```python
from build123d import *

# Parameters (mm, degrees)
PAD007_DEPTH    = 2
PAD008_DEPTH    = 1
SKETCH021_W     = 20.3
SKETCH021_H     = 23.4
POCKET008_DEPTH = 0.6
PAD009_DEPTH    = 3
SKETCH024_W     = 7.2
SKETCH024_H     = 1.2
POCKET010_DEPTH = 1.2
FILLET002_R     = 0.9


with BuildPart() as part:
    # Sketch019 → Pad007 (new body)
    with BuildSketch(Plane.XY):
        with BuildLine():
            Line((-13.864971, -3.085), (14.264998, -3.085))
            ThreePointArc((14.264998, -3.085), (18.224807, -1.444793), (19.865014, 2.515016))
            Line((19.865014, 2.515016), (19.865014, 23.284984))
            ThreePointArc((19.865014, 23.284984), (18.224807, 27.244793), (14.264998, 28.885))
            Line((14.264998, 28.885), (-13.864971, 28.885))
            ThreePointArc((-13.864971, 28.885), (-17.82478, 27.244793), (-19.464986, 23.284984))
            Line((-19.464986, 23.284984), (-19.464986, 2.515016))
            ThreePointArc((-19.464986, 2.515016), (-17.82478, -1.444793), (-13.864971, -3.085))
        make_face()
        with BuildLine():
            Line((-18.464986, 23.284984), (-18.464986, 2.515016))
            ThreePointArc((-18.464986, 2.515016), (-17.117673, -0.737687), (-13.864971, -2.085))
            Line((-13.864971, -2.085), (14.264998, -2.085))
            ThreePointArc((14.264998, -2.085), (17.5177, -0.737687), (18.865014, 2.515016))
            Line((18.865014, 2.515016), (18.865014, 23.284984))
            ThreePointArc((18.865014, 23.284984), (17.5177, 26.537687), (14.264998, 27.885))
            Line((14.264998, 27.885), (-13.864971, 27.885))
            ThreePointArc((-13.864971, 27.885), (-17.117673, 26.537687), (-18.464986, 23.284984))
        make_face(mode=Mode.SUBTRACT)
    extrude(amount=PAD007_DEPTH)

    # Sketch020 → Pad008 (join)
    with BuildSketch(Plane.XY):
        with BuildLine():
            Line((-20.964986, 23.284984), (-20.964986, 2.515016))
            ThreePointArc((-20.964986, 2.515016), (-18.88544, -2.505454), (-13.864971, -4.585))
            Line((-13.864971, -4.585), (14.264998, -4.585))
            ThreePointArc((14.264998, -4.585), (19.285467, -2.505454), (21.365014, 2.515016))
            Line((21.365014, 2.515016), (21.365014, 23.284984))
            ThreePointArc((21.365014, 23.284984), (19.285467, 28.305454), (14.264998, 30.385))
            Line((14.264998, 30.385), (-13.864971, 30.385))
            ThreePointArc((-13.864971, 30.385), (-18.88544, 28.305454), (-20.964986, 23.284984))
        make_face()
    extrude(amount=-PAD008_DEPTH)

    # Sketch021 → Pocket008 (cut)
    with BuildSketch(Plane.XY):
        with Locations((8.55, 12.7)):
            Rectangle(SKETCH021_W, SKETCH021_H)
    extrude(amount=-POCKET008_DEPTH, mode=Mode.SUBTRACT)

    # Sketch023 → Pad009 (join)
    with BuildSketch(Plane.XZ):
        Polygon((-13.864971, 0), (14.264998, 0), (14.264998, 8.25), (12.364998, 8.25), (12.364998, 4.75), (6.164998, 4.75), (6.164998, 8.25), (3.1, 8.25), (3.1, 4.75), (-3.1, 4.75), (-3.1, 8.25), (-5.764971, 8.25), (-5.764971, 4.75), (-11.964971, 4.75), (-11.964971, 8.25), (-13.864971, 8.25), align=None)
    extrude(amount=PAD009_DEPTH)

    # Sketch024 → Pocket010 (cut)
    with BuildSketch(Plane.XZ):
        with Locations((-8.864971, 6.5)):
            Rectangle(SKETCH024_W, SKETCH024_H)
        with Locations((0, 6.5)):
            Rectangle(SKETCH024_W, SKETCH024_H)
        with Locations((9.264998, 6.5)):
            Rectangle(SKETCH024_W, SKETCH024_H)
    extrude(amount=POCKET010_DEPTH, mode=Mode.SUBTRACT)

    # Fillet002
    fillet002_edges = [part.edges().sort_by_distance(p)[0] for p in [
        (-20.964986, 12.9, -1),
        (-18.88544, 28.305454, -1),
        (0.200014, 30.385, -1),
        (19.285467, 28.305454, -1),
        (21.365014, 12.9, -1),
        (19.285467, -2.505454, -1),
        (0.200014, -4.585, -1),
        (-18.88544, -2.505454, -1),
    ]]
    fillet(fillet002_edges, radius=FILLET002_R)


with BuildPart() as part_1:
    # Body004 placement: moved
    add(part.part.moved(Location((0, 0, 0.9))))


solid = part_1.part
```
The listing builds one solid part. Answer for the finished solid, in the listing's coordinates (mm). A direction names the side the tool comes from. Coordinates: 2 decimals unless noted, no trailing zeros. Loops run counter-clockwise (first coordinate to the right, second up) from the corner with the lowest first, then second, coordinate; pieces in that order, holes last. Notation, with made-up numbers: (73.25, 8.25) -> (104.25, 8.25) arc R19 ccw to (104.25, 44.25) -> close; hole circle Ø1 at (-25.5, 3). An arc over 180 degrees is marked (long way). Return JSON: item names as keys, results as strings. Group by question number.
(1) A cutting plane is placed at D-D on z = 5. Write down the section's boundary in (x, y) (3 decimals), and give its area (3 significant figures).
(2) Find the intervals of material crossed by probe 1 along X at (y, z) = (18, 1.75); probe 2 along X at (y, z) = (-1, 2.25) (3 decimals); probe 3 along Z at (x, y) = (10.5, 25), in increasing order. Write a range as from..to.
(3) A cutting plane is placed at B-B on z = 2. Write down the section's boundary in (x, y) (3 decimals), and give its area (3 significant figures).
(4) A cutting plane is placed at A-A on y = 4. Write down the section's boundary in (x, z), and give its area (3 significant figures).
(5) Which of the six approach directions +Z, -Z, +X, -X, +Y, -Y give full straight-line access (tool end or side, diameter ignored) to faces 1 (the flat face through (0, -3, 5)), 2 (the flat face through (19.865, 13, 2)), 3 (the flat face through (0, -4, 0.9)), 4 (the cylindrical face through (18.18, -1.49, 1.89))?
(6) Determine the mould class of faces 5 (the flat face through (-5.265, -1, 7)), 6 (the cylindrical face through (0.4, -4.33, 0.17)), 7 (the flat face through (3.6, -1, 7)), 8 (the cylindrical face through (-17.87, -1.4, 1.89)) for opening direction X: released by +X, released by -X, zero draft, split by the parting line, or undercut.
(7) A cutting plane is placed at C-C on x = -6.5. Write down the section's boundary in (y, z) (3 decimals).
(8) Given pin 1 Ø1.3 at (y, z) = (-1, 7.5) entering from +X (3 decimals); pin 2 Ø4 at (x, z) = (12.5, 8) entering from -Y; pin 3 Ø2 at (y, z) = (8, 2) entering from -X (3 decimals); pin 4 Ø0.6 at (x, y) = (-3, -0.5) entering from +Z, each flat-ended and moving along its own axis, determine where each tip first touches the part or whether it passes through.
The answers:
{
 "1": {"outline": "(-13.865, -3) -> (14.265, -3) -> (14.265, 0) -> (-13.865, 0) -> close", "area": "84.4 mm^2"},
 "2": {"probe 1": "x = -19.46..-18.46, 18.87..19.87", "probe 2": "x = -18.224..-16.832, -13.865..14.265, 17.232..18.624", "probe 3": "z = -0.1..0.9"},
 "3": {"outline": "(-19.465, 2.515) arc R5.6 ccw to (-13.865, -3.085) -> (14.265, -3.085) arc R5.6 ccw to (19.865, 2.515) -> (19.865, 23.285) arc R5.6 ccw to (14.265, 28.885) -> (-13.865, 28.885) arc R5.6 ccw to (-19.465, 23.285) -> close; hole (-18.465, 2.515) arc R4.6 ccw to (-13.865, -2.085) -> (-13.865, 0) -> (14.265, 0) -> (14.265, -2.085) arc R4.6 ccw to (18.865, 2.515) -> (18.865, 23.285) arc R4.6 ccw to (14.265, 27.885) -> (-13.865, 27.885) arc R4.6 ccw to (-18.465, 23.285) -> close", "area": "188 mm^2"},
 "4": {"outline": "(-20.96, 0.8) arc R0.9 ccw to (-20.06, -0.1) -> (20.47, -0.1) arc R0.9 ccw to (21.37, 0.8) -> (21.37, 0.9) -> (19.87, 0.9) -> (19.87, 2.9) -> (18.87, 2.9) -> (18.87, 0.9) -> (18.7, 0.9) -> (18.7, 0.3) -> (-1.6, 0.3) -> (-1.6, 0.9) -> (-18.46, 0.9) -> (-18.46, 2.9) -> (-19.46, 2.9) -> (-19.46, 0.9) -> (-20.96, 0.9) -> close", "area": "33.8 mm^2"},
 "5": {"face 1": "+Z, +X, -X, -Y", "face 2": "+Z, +X, +Y, -Y", "face 3": "+Z", "face 4": "+Z, +X, -Y"},
 "6": {"face 5": "undercut", "face 6": "zero draft", "face 7": "undercut", "face 8": "released by -X"},
 "7": {"outline": "(-4.585, 0.8) arc R0.9 ccw to (-3.685, -0.1) -> (29.485, -0.1) arc R0.9 ccw to (30.385, 0.8) -> (30.385, 0.9) -> (28.885, 0.9) -> (28.885, 2.9) -> (27.885, 2.9) -> (27.885, 0.9) -> (0, 0.9) -> (0, 5.65) -> (-3, 5.65) -> (-3, 2.9) -> (-3.085, 2.9) -> (-3.085, 0.9) -> (-4.585, 0.9) -> close"},
 "8": {"pin 1": "stops at x = 14.265", "pin 2": "stops at y = -3", "pin 3": "stops at x = -19.465", "pin 4": "stops at z = 9.15"}
}
